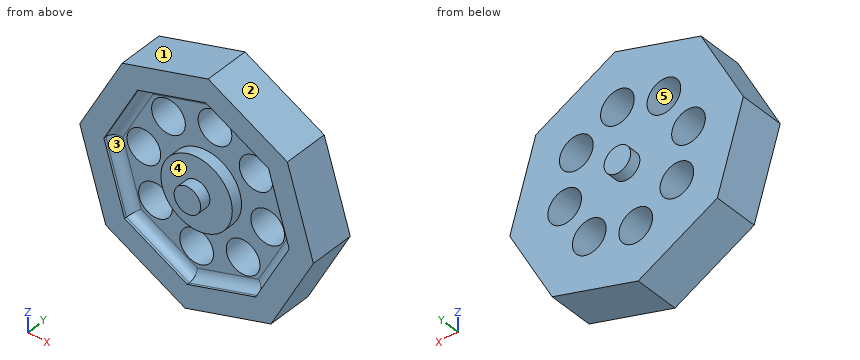
```python
from build123d import *

# Parameters (mm, degrees)
F0_R     = 7.5
F1_DEPTH = 12.7
F2_DEPTH = 19.05
F3_R     = 9.525
F3_R_2   = 20.2
F4_DEPTH = 6.35
F5_DEPTH = 31.751
F6_R     = 5.08


with BuildPart() as f1:
    # F0 (on Front) → F1 (new body, symmetric)
    with BuildSketch(Plane.XZ):
        Polygon((66.049778, -6.546358), (51.333221, 42.075272), (6.546358, 66.049778), (-42.075272, 51.333221), (-66.049778, 6.546358), (-51.333221, -42.075272), (-6.546358, -66.049778), (42.075272, -51.333221), align=None)
        Circle(F0_R, mode=Mode.SUBTRACT)
    extrude(amount=F1_DEPTH, both=True)

    # F0 (on Front) → F2 (join, symmetric)
    with BuildSketch(Plane.XZ):
        Circle(F0_R)
    extrude(amount=F2_DEPTH, both=True)

    # F3 (on face) → F4 (cut)
    with BuildSketch(Plane.XZ.offset(12.7)):
        Polygon((-5.190563, -52.370421), (33.361198, -40.701763), (52.370421, -5.190563), (40.701763, 33.361198), (5.190563, 52.370421), (-33.361198, 40.701763), (-52.370421, 5.190563), (-40.701763, -33.361198), align=None)
        with Locations((-5.190563, -35.008609)):
            Circle(F3_R, mode=Mode.SUBTRACT)
        with Locations((-28.425107, -21.084543)):
            Circle(F3_R, mode=Mode.SUBTRACT)
        with Locations((21.084543, -28.425107)):
            Circle(F3_R, mode=Mode.SUBTRACT)
        Circle(F3_R_2, mode=Mode.SUBTRACT)
        with Locations((35.008609, -5.190563)):
            Circle(F3_R, mode=Mode.SUBTRACT)
        with Locations((-35.008609, 5.190563)):
            Circle(F3_R, mode=Mode.SUBTRACT)
        with Locations((-21.084543, 28.425107)):
            Circle(F3_R, mode=Mode.SUBTRACT)
        with Locations((28.425107, 21.084543)):
            Circle(F3_R, mode=Mode.SUBTRACT)
        with Locations((5.190563, 35.008609)):
            Circle(F3_R, mode=Mode.SUBTRACT)
    extrude(amount=-F4_DEPTH, mode=Mode.SUBTRACT)

    # F3 (on face) → F5 (cut, through all)
    with BuildSketch(Plane.XZ.offset(12.7)):
        with Locations((-35.008609, 5.190563)):
            Circle(F3_R)
        with Locations((-21.084543, 28.425107)):
            Circle(F3_R)
        with Locations((5.190563, 35.008609)):
            Circle(F3_R)
        with Locations((28.425107, 21.084543)):
            Circle(F3_R)
        with Locations((21.084543, -28.425107)):
            Circle(F3_R)
        with Locations((-28.425107, -21.084543)):
            Circle(F3_R)
        with Locations((35.008609, -5.190563)):
            Circle(F3_R)
        with Locations((-5.190563, -35.008609)):
            Circle(F3_R)
    extrude(amount=-F5_DEPTH, mode=Mode.SUBTRACT)

    # F6
    f6_edges = [f1.edges().sort_by_distance(p)[0] for p in [
        (-14.085317, -6.35, 46.536092),
        (-42.86581, -6.35, 22.946163),
        (-46.536092, -6.35, -14.085317),
        (-22.946163, -6.35, -42.86581),
        (22.946163, -6.35, 42.86581),
        (46.536092, -6.35, 14.085317),
        (42.86581, -6.35, -22.946163),
        (14.085317, -6.35, -46.536092),
    ]]
    fillet(f6_edges, radius=F6_R)


solid = f1.part
```
Verification items for the finished model (mm, model axes). Face numbers are marked on the shaded views. A direction names the side the tool comes from. Coordinates: 2 decimals unless noted, no trailing zeros. Write each loop counter-clockwise with the first axis right and the second up, starting at its lowest first coordinate (ties: lowest second). Pieces come first, ordered by that corner, then holes. Notation, with made-up numbers: M 45,27 L 95,27 A17 cw 95,41 Z; hole C 20.5,-34 d3. An arc over 180 degrees is marked long. Answer as a JSON object with one key per item and string values. Group by question number.
(1) Tool access check on the marked faces 4 and 5. Record the directions out of +Z, -Z, +X, -X, +Y, -Y that give a thin tool (end or side, any length) a straight path to the whole face; none if there is none.
(2) Gauge pin test, flat ends, axial feed: pin 1 (22 mm diameter, centred on x = -35.01, z = 5.19, fed in from +Y); pin 2 (8 mm diameter, centred on x = -15, y = -11.5, fed in from -Z); pin 3 (1.5 mm diameter, centred on y = 12, z = -44, fed in from +X); pin 4 (15 mm diameter, centred on x = 35.01, z = -5.19, fed in from +Y). Record the tip position at first contact, or that the pin passes through.
(3) Cross-section at A-A, the plane y = -8.5. Record the cut outline in (x, z).
(4) Material ranges on line 1 (Z direction, x = 32.5, y = 4.5); line 2 (X direction, y = 0.5, z = 25); line 3 (X direction, y = 8, z = 13), recorded low to high.
(5) Cross-section at B-B, the plane z = 0. State how many separate pieces and enclosed holes the cut face has, and give its area (3 significant figures).
(6) Cross-section at D-D, the plane x = 55.5. Record the cut outline in (y, z), and give its area (3 significant figures).
(7) Release check for a two-part mould opening along X. For the marked faces 1, 2 and 3 record: +X half, -X half, draft (parallel to the pull), parting line (faces both ways), or undercut.
Reply:
{
 "1": {"face 4": "-Y", "face 5": "+Y, -Y"},
 "2": {"pin 1": "y = 12.7", "pin 2": "z = -63.67", "pin 3": "x = 46.4", "pin 4": "through"},
 "3": {"outline": "M -66.05,6.55 L -51.33,-42.08 L -6.55,-66.05 L 42.08,-51.33 L 66.05,-6.55 L 51.33,42.08 L 6.55,66.05 L -42.08,51.33 Z; C 0,0 d40.4; hole M -51.37,5.09 L -39.92,-32.72 L -5.09,-51.37 L 32.72,-39.92 L 51.37,-5.09 L 39.92,32.72 L 5.09,51.37 L -32.72,39.92 Z"},
 "4": {"line 1": "-54.23 to -14.38, 4 to 12.48, 29.69 to 52.16", "line 2": "-56.17 to -29.97, -12.2 to 19.74, 37.11 to 56.5", "line 3": "-62.6 to -40.46, -29.56 to 23.39, 33.46 to 60.13"},
 "5": {"separate pieces": "3", "enclosed holes": "0", "area": "2,460 mm²"},
 "6": {"outline": "M -12.7,-26.25 L 12.7,-26.25 L 12.7,28.31 L -12.7,28.31 Z", "area": "1,390 mm²"},
 "7": {"face 1": "-X half", "face 2": "+X half", "face 3": "undercut"}
}
